Work out the finished part from the listing and answer in its coordinate system (mm). A direction names the side the tool comes from. Round coordinates to 2 decimals unless told otherwise and drop trailing zeros. Order: outer loops, then holes, each group sorted by start corner. A loop starts at its lowest first (then second) coordinate and runs counter-clockwise, first axis right, second up. Notation, with made-up numbers: M 59,85 L 73,85 A20 ccw 73,108 Z; hole C -22.75,-37 d11. An arc over 180 degrees is marked long. Return JSON: item names as keys, results as strings.
from build123d import *

# Parameters (mm, degrees)
EXTRUSION1_DEPTH = 50
EXTRUSION2_REACH = 21.092
ESQUISSE3_R      = 2.5
EXTRUSION3_REACH = 29.642
ESQUISSE4_R      = 1.5


with BuildPart() as part:
    # Esquisse1 → Extrusion1 (new body)
    with BuildSketch(Plane(origin=(0, 0, 0), x_dir=(1, 0, 0), z_dir=(0, 1, 0))):
        Polygon((0, 0), (0, 20), (17.67766953, 37.67766953), (19.091883092, 36.263455967), (2, 19.171572875), (2, 0), align=None)
    extrude(amount=EXTRUSION1_DEPTH)

    # Esquisse3 → Extrusion2 (cut, up to next)
    with BuildSketch(Plane.ZY, mode=Mode.PRIVATE) as extrusion2_sk1:
        with Locations((-10, 5)):
            Circle(ESQUISSE3_R)
    extrusion2_tool1 = extrude(extrusion2_sk1.sketch, amount=-EXTRUSION2_REACH, mode=Mode.PRIVATE) & part.part
    add(extrusion2_tool1.solids().sort_by_distance((0, 5, -10))[0], mode=Mode.SUBTRACT)
    # Esquisse3 → Extrusion2 (cut, up to next)
    with BuildSketch(Plane.ZY, mode=Mode.PRIVATE) as extrusion2_sk2:
        with Locations((-10, 45)):
            Circle(ESQUISSE3_R)
    extrusion2_tool2 = extrude(extrusion2_sk2.sketch, amount=-EXTRUSION2_REACH, mode=Mode.PRIVATE) & part.part
    add(extrusion2_tool2.solids().sort_by_distance((0, 45, -10))[0], mode=Mode.SUBTRACT)

    # Esquisse4 → Extrusion3 (cut, up to next)
    with BuildSketch(Plane(origin=(-10, 0, -10), x_dir=(-0.707106781, 0, 0.707106781), z_dir=(-0.707106781, 0, -0.707106781)), mode=Mode.PRIVATE) as extrusion3_sk1:
        with Locations((-26.642135624, 43.5)):
            Circle(ESQUISSE4_R)
    extrusion3_tool1 = extrude(extrusion3_sk1.sketch, amount=-EXTRUSION3_REACH, mode=Mode.PRIVATE) & part.part
    add(extrusion3_tool1.solids().sort_by_distance((8.838835, 43.5, -28.838835))[0], mode=Mode.SUBTRACT)
    # Esquisse4 → Extrusion3 (cut, up to next)
    with BuildSketch(Plane(origin=(-10, 0, -10), x_dir=(-0.707106781, 0, 0.707106781), z_dir=(-0.707106781, 0, -0.707106781)), mode=Mode.PRIVATE) as extrusion3_sk2:
        with Locations((-26.642135624, 6.5)):
            Circle(ESQUISSE4_R)
    extrusion3_tool2 = extrude(extrusion3_sk2.sketch, amount=-EXTRUSION3_REACH, mode=Mode.PRIVATE) & part.part
    add(extrusion3_tool2.solids().sort_by_distance((8.838835, 6.5, -28.838835))[0], mode=Mode.SUBTRACT)


solid = part.part
Item 1: Find section B-B (y = 10). Determine the outline of the cut face in (x, z), plus the area to 3 significant figures.
Output:
{"outline": "M 0,-20 L 17.68,-37.68 L 19.09,-36.26 L 2,-19.17 L 2,0 L 0,0 Z", "area": "88.3 mm^2"}
Item 2: Consider line 1 along Y through (x, z) = (0.6, -10); line 2 along X through (y, z) = (22.5, -10); line 3 along Z through (x, y) = (17, 42.5). Determine where each line is inside the solid, lowest interval first. Write a range as [from, to].
Output:
{"line 1": "y = [0, 2.5], [7.5, 42.5], [47.5, 50]", "line 2": "x = [0, 2]", "line 3": "z = [-37, -34.17]"}
Item 3: Which of the six approach directions +Z, -Z, +X, -X, +Y, -Y give full straight-line access (tool end or side, diameter ignored) to faces 5 (the flat face through (2, 25, -10)), 6 (the flat face through (4, 50, -22))?
Output:
{"face 5": "+Z, +X, +Y, -Y", "face 6": "+Z, -Z, +X, -X, +Y"}
Item 4: Find section C-C (x = 16.25). Determine the outline of the cut face in (y, z), plus the area to 3 significant figures.
Output:
{"outline": "M 0,-36.25 L 50,-36.25 L 50,-33.42 L 0,-33.42 Z", "area": "141 mm^2"}
Item 5: The mould has two halves that part along X. Classify faces 1 (the cylindrical face through (8.556, 5.925, -27.162)), 2 (the cylindrical face through (9.766, 42.036, -28.372)), 3 (the flat face through (1, 25, 0)), 4 (the flat face through (10.67, 24.65, -27.84)): pulls with the +X half, pulls with the -X half, needs draft (parallel to the pull), parting line crosses it, or undercut.
Output:
{"face 1": "undercut", "face 2": "undercut", "face 3": "needs draft", "face 4": "pulls with the +X half"}
Item 6: Each of these flat-tipped pins is pushed along its axis until it touches: pin 1 (3 mm diameter, centred on x = 12.5, y = 17.5, fed in from +Z); pin 2 (4 mm diameter, centred on y = 23, z = -9.5, fed in from +X); pin 3 (15.5 mm diameter, centred on y = 24, z = -13.5, fed in from +X). Where does it stop, or does it pass through?
Output:
{"pin 1": "stops at z = -28.17", "pin 2": "stops at x = 2", "pin 3": "stops at x = 4.08"}
Item 7: Find section A-A (z = -10). Determine the outline of the cut face in (x, y).
Output:
{"outline": "M 0,0 L 2,0 L 2,2.5 L 0,2.5 Z; M 0,7.5 L 2,7.5 L 2,42.5 L 0,42.5 Z; M 0,47.5 L 2,47.5 L 2,50 L 0,50 Z"}
Item 8: Find section D-D (z = -32.5). Determine the outline of the cut face in (x, y), plus the area to 3 significant figures.
Output:
{"outline": "M 12.5,0 L 15.33,0 L 15.33,50 L 12.5,50 Z", "area": "141 mm^2"}
